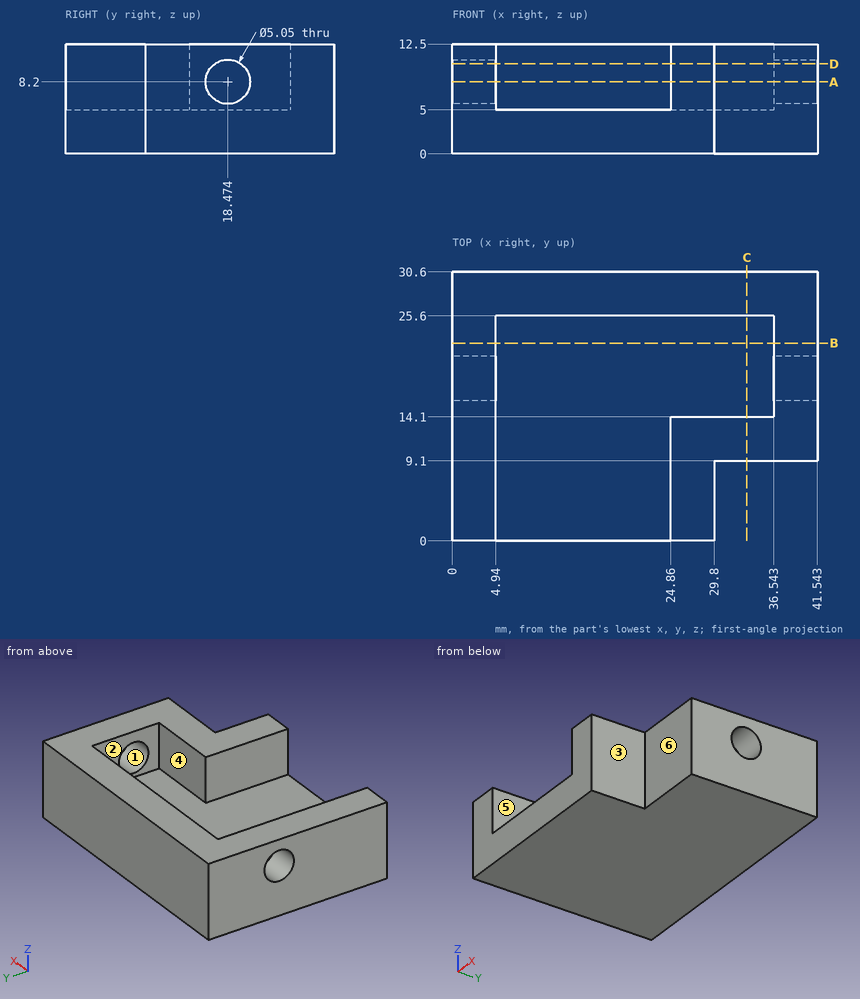
Design review of the part shown in the three views and the two pictorial views. Dimensions are in mm from the part's minimum x, y and z. A direction names the side the tool comes from. Round coordinates to 2 decimals unless told otherwise and drop trailing zeros. Write each loop counter-clockwise with the first axis right and the second up, starting at its lowest first coordinate (ties: lowest second). Pieces come first, ordered by that corner, then holes. Notation, with made-up numbers: (84.25, -5) -> (115.25, -5) arc R20 ccw to (115.25, 9) -> close; hole circle Ø7 at (35, 49). An arc over 180 degrees is marked (long way). Use one line per item in the form item = value.
1) Take a section at B-B, the plane y = 22.5. Write out the cut boundary in (x, z), and give its area (3 significant figures).
Found:
outline = (0, 0) -> (41.54, 0) -> (41.54, 12.5) -> (36.54, 12.5) -> (36.54, 5) -> (4.94, 5) -> (4.94, 12.5) -> (0, 12.5) -> close
area = 282 mm2
2) Tool access review of the marked faces 4, 5 and 6: name each direction out of +Z, -Z, +X, -X, +Y, -Y from which nothing blocks a thin tool from reaching the whole face with its end or side.
Found:
face_4 = +Z
face_5 = +Z, -Y
face_6 = +Z, -Z, +X, -Y
3) Take a section at C-C, the plane x = 33.5. Write out the cut boundary in (y, z).
Found:
outline = (9.1, 0) -> (30.6, 0) -> (30.6, 12.5) -> (25.6, 12.5) -> (25.6, 5) -> (14.1, 5) -> (14.1, 12.5) -> (9.1, 12.5) -> close
4) Mouldability with a two-part tool opening along X and no side actions: class the marked faces 1, 2 and 3 as +X half, -X half, draft (parallel to the pull), parting line (faces both ways), or undercut.
Found:
face_1 = draft
face_2 = undercut
face_3 = +X half
5) Take a section at D-D, the plane z = 10.25. Write out the cut boundary in (x, y).
Found:
outline = (0, 0) -> (4.94, 0) -> (4.94, 17) -> (0, 17) -> close; (0, 19.95) -> (4.94, 19.95) -> (4.94, 25.6) -> (36.54, 25.6) -> (36.54, 19.95) -> (41.54, 19.95) -> (41.54, 30.6) -> (0, 30.6) -> close; (24.86, 0) -> (29.8, 0) -> (29.8, 9.1) -> (41.54, 9.1) -> (41.54, 17) -> (36.54, 17) -> (36.54, 14.1) -> (24.86, 14.1) -> close
6) Clearance check with flat-ended pins moving along their axes: pin 1 (2.5 mm diameter, centred on y = 3.5, z = 6, fed in from +X); pin 2 (12 mm diameter, centred on x = 12, y = 7.5, fed in from +Z). State where each tip first meets the part, or that it passes through.
Found:
pin_1 = 29.8
pin_2 = 5
7) Take a section at A-A, the plane z = 8.2. Write out the cut boundary in (x, y), and give its area (3 significant figures).
Found:
outline = (0, 0) -> (4.94, 0) -> (4.94, 15.95) -> (0, 15.95) -> close; (0, 21) -> (4.94, 21) -> (4.94, 25.6) -> (36.54, 25.6) -> (36.54, 21) -> (41.54, 21) -> (41.54, 30.6) -> (0, 30.6) -> close; (24.86, 0) -> (29.8, 0) -> (29.8, 9.1) -> (41.54, 9.1) -> (41.54, 15.95) -> (36.54, 15.95) -> (36.54, 14.1) -> (24.86, 14.1) -> close
area = 470 mm2
8) To check wall thickness, follow L1, parallel to X at y = 18, z = 5.5; L2, parallel to Y at x = 3.1, z = 8.2; L3, parallel to X at y = 8, z = 6. State the ranges of each line that lie inside material, in increasing order. Write a range as from..to.
Found:
L1 = 0..4.94, 36.54..41.54
L2 = 0..15.95, 21..30.6
L3 = 0..4.94, 24.86..29.8
